Can you work these out from the model? Positions are in its coordinate system, mm. Give positions to 0.01 mm unless a question says otherwise; leave off trailing zeros. Write each loop counter-clockwise with the first axis right and the second up, starting at its lowest first coordinate (ties: lowest second). Pieces come first, ordered by that corner, then holes.
```python
from build123d import *

# Parameters (mm, degrees)
BOSS_EXTRUDE1_DEPTH = 5.9944
SKETCH2_R           = 5.08
CUT_EXTRUDE1_DEPTH  = 369.278830147
CUT_EXTRUDE2_DEPTH  = 1.27
FILLET1_R           = 6.35


with BuildPart() as part:
    # Sketch1 → Boss-Extrude1 (new body)
    with BuildSketch(Plane(origin=(0, 0, 0), x_dir=(1, 0, 0), z_dir=(0, 1, 0))):
        Polygon((-67.6275, 0), (67.6275, 0), (95.613826947, -355.6), (-95.613826947, -355.6), align=None)
    extrude(amount=BOSS_EXTRUDE1_DEPTH)

    # Sketch2 → Cut-Extrude1 (cut, through all)
    with BuildSketch(Plane(origin=(0, 5.9944, 0), x_dir=(1, 0, 0), z_dir=(0, 1, 0))):
        with Locations(Location((0, -101.6, 0), (0, 0, 270))):
            Circle(SKETCH2_R)
    extrude(amount=-CUT_EXTRUDE1_DEPTH, mode=Mode.SUBTRACT)

    # Sketch3 → Cut-Extrude2 (cut)
    # profile 1 of 2: a face of its own
    with BuildSketch(Plane(origin=(0, 5.9944, 0), x_dir=(1, 0, 0), z_dir=(0, 1, 0))):
        Polygon((-0.64745098, -123.339411765), (-2.041960784, -123.339411765), (-2.041960784, -125.73), (-2.838823529, -125.73), (-2.838823529, -123.339411765), (-7.420784314, -123.339411765), (-7.420784314, -122.54254902), (-2.676960784, -115.769215686), (-2.041960784, -115.769215686), (-2.041960784, -122.54254902), (-0.64745098, -122.54254902), align=None)
        Polygon((-2.838823529, -122.54254902), (-2.838823529, -117.185514706), (-6.589681373, -122.54254902), align=None, mode=Mode.SUBTRACT)
    # profile 2 of 2: a face of its own
    with BuildSketch(Plane(origin=(0, 5.9944, 0), x_dir=(1, 0, 0), z_dir=(0, 1, 0))):
        with BuildLine():
            add(Edge.make_bspline(
                [(7.321176471, -120.755833333), (7.318828398, -120.964435203), (7.314268428, -121.369541156), (7.278053355, -121.956745016), (7.212590307, -122.503235643), (7.123658685, -123.008755237), (7.008266172, -123.474678786), (6.871087333, -123.902056716), (6.702092819, -124.287425995), (6.508215245, -124.632617465), (6.291747836, -124.939879658), (6.045192851, -125.205053414), (5.774903263, -125.430333986), (5.47658793, -125.612983557), (5.154255704, -125.75891836), (4.803074469, -125.854617169), (4.428855706, -125.921386338), (4.17035965, -125.926554175), (4.037230392, -125.929215686)],
                knots=[0, 0, 0, 0, 1.444951835, 2.806104229, 4.07292158, 5.255788138, 6.359234241, 7.395665143, 8.361159583, 9.268708362, 10.134304339, 10.95819393, 11.769860228, 12.563733626, 13.374508403, 14.211708464, 15.079003648, 16, 16, 16, 16], degree=3))
            add(Edge.make_bspline(
                [(4.037230392, -125.929215686), (3.904173743, -125.926129436), (3.644961099, -125.920116997), (3.27017657, -125.859085315), (2.920411161, -125.763594373), (2.59640029, -125.625895969), (2.300139806, -125.446021212), (2.024069589, -125.233082993), (1.778627689, -124.975727427), (1.560171839, -124.679785297), (1.365195047, -124.347714828), (1.20253453, -123.973246068), (1.058366082, -123.562916679), (0.945634561, -123.112374896), (0.854092493, -122.625055928), (0.795691583, -122.097466824), (0.752427723, -121.531621273), (0.748884772, -121.140869167), (0.747058824, -120.939485294)],
                knots=[0, 0, 0, 0, 0.942187573, 1.835510922, 2.682899358, 3.50644207, 4.321041037, 5.132947656, 5.970162763, 6.831912057, 7.734836617, 8.692673853, 9.720484412, 10.813675431, 11.980358204, 13.231647047, 14.573260056, 16, 16, 16, 16], degree=3))
            add(Edge.make_bspline(
                [(0.747058824, -120.939485294), (0.749189738, -120.709081181), (0.753301018, -120.264550974), (0.791785956, -119.623892076), (0.848921011, -119.033607435), (0.931327178, -118.493626742), (1.041809864, -118.002956136), (1.18209133, -117.562748274), (1.344352733, -117.168906906), (1.542969603, -116.826611164), (1.76640963, -116.527719309), (2.011736134, -116.265404707), (2.288722816, -116.05041743), (2.588716504, -115.873144616), (2.914180915, -115.735469097), (3.266151279, -115.640569114), (3.642854433, -115.578856283), (3.90312556, -115.573011518), (4.037230392, -115.57)],
                knots=[0, 0, 0, 0, 1.545108237, 2.981054794, 4.302900454, 5.52134946, 6.64223763, 7.672189641, 8.617001291, 9.493094031, 10.318410963, 11.115795503, 11.893970542, 12.661367534, 13.447190288, 14.255881535, 15.101342067, 16, 16, 16, 16], degree=3))
            add(Edge.make_bspline(
                [(4.037230392, -115.57), (4.170238627, -115.57448963), (4.428282356, -115.583199774), (4.804192318, -115.642018007), (5.152618043, -115.745772402), (5.478653289, -115.884356647), (5.772542755, -116.073295118), (6.047681503, -116.293496105), (6.289327541, -116.562467111), (6.510315761, -116.867199073), (6.701841879, -117.215226558), (6.869820244, -117.601739646), (7.009467972, -118.029371708), (7.123413066, -118.496780378), (7.21266615, -119.005311375), (7.277684225, -119.552884468), (7.314472673, -120.141074122), (7.318890361, -120.546189931), (7.321176471, -120.755833333)],
                knots=[0, 0, 0, 0, 0.919968977, 1.784793451, 2.622728724, 3.429378823, 4.225844794, 5.031728358, 5.85964663, 6.718105312, 7.630541726, 8.601153045, 9.629202519, 10.737948011, 11.926092541, 13.198121829, 14.550055913, 16, 16, 16, 16], degree=3))
        make_face()
        with BuildLine():
            add(Edge.make_bspline(
                [(6.524313725, -120.768284314), (6.522566947, -120.59082563), (6.519183425, -120.247086842), (6.491882586, -119.747351272), (6.442379883, -119.282006526), (6.374689104, -118.850591154), (6.287787289, -118.454473729), (6.184085269, -118.091152232), (6.054789642, -117.764549081), (5.914753741, -117.468482457), (5.746577036, -117.21145005), (5.563889756, -116.983709924), (5.356631682, -116.79434266), (5.134096525, -116.633668508), (4.887159424, -116.51702345), (4.624573174, -116.42744118), (4.339914631, -116.378499272), (4.144272117, -116.370819959), (4.043455882, -116.366862745)],
                knots=[0, 0, 0, 0, 1.502278276, 2.909924168, 4.234983773, 5.462469173, 6.604815465, 7.666614396, 8.656743616, 9.57599474, 10.43362925, 11.251287335, 12.040715275, 12.803499886, 13.565626727, 14.343386511, 15.146333119, 16, 16, 16, 16], degree=3))
            add(Edge.make_bspline(
                [(4.043455882, -116.366862745), (3.938447052, -116.369409337), (3.734422845, -116.374357173), (3.43835687, -116.425549656), (3.163244621, -116.509328168), (2.90892764, -116.62546025), (2.673837753, -116.772323146), (2.465862577, -116.959962497), (2.272440236, -117.175944485), (2.105615234, -117.430931462), (1.958401995, -117.71853329), (1.838162718, -118.042916058), (1.738143905, -118.401926091), (1.665875136, -118.800267442), (1.610637384, -119.239896883), (1.570198504, -119.724849093), (1.550557152, -120.257632824), (1.546194025, -120.628198528), (1.543921569, -120.82120098)],
                knots=[0, 0, 0, 0, 0.869467109, 1.689308758, 2.480750345, 3.246411928, 4.000153033, 4.767743238, 5.559605047, 6.396624794, 7.284891774, 8.231849658, 9.258192498, 10.369472511, 11.583108734, 12.929054675, 14.400553601, 16, 16, 16, 16], degree=3))
            add(Edge.make_bspline(
                [(1.543921569, -120.82120098), (1.544614632, -120.988289367), (1.54595406, -121.311207558), (1.570315432, -121.778131708), (1.598441181, -122.210377927), (1.645028029, -122.609499828), (1.709082826, -122.979104893), (1.796740701, -123.322117953), (1.902442711, -123.64204798), (2.027679077, -123.937897338), (2.18133626, -124.206925847), (2.364747317, -124.444835267), (2.580966733, -124.649942715), (2.82339308, -124.825742486), (3.097933318, -124.96336255), (3.398653863, -125.062824592), (3.726651153, -125.123356927), (3.95395607, -125.129287098), (4.071470588, -125.132352941)],
                knots=[0, 0, 0, 0, 1.411809826, 2.728490499, 3.95043818, 5.071756233, 6.122676174, 7.117949067, 8.060697316, 8.967954545, 9.828234386, 10.671864258, 11.496693245, 12.338635446, 13.193491276, 14.080783746, 15.007783125, 16, 16, 16, 16], degree=3))
            add(Edge.make_bspline(
                [(4.071470588, -125.132352941), (4.170329033, -125.130072963), (4.364367231, -125.125597848), (4.644218388, -125.069712213), (4.907756322, -124.987576413), (5.148049832, -124.862984482), (5.372323269, -124.710857365), (5.572547405, -124.519087844), (5.758725654, -124.297778208), (5.918122592, -124.036648789), (6.062406119, -123.745178799), (6.186127809, -123.4196766), (6.291039197, -123.06045838), (6.37874373, -122.667596662), (6.4407328, -122.240695517), (6.492645246, -121.781020892), (6.51900758, -121.286348012), (6.522506852, -120.944697746), (6.524313725, -120.768284314)],
                knots=[0, 0, 0, 0, 0.843506666, 1.655625022, 2.429524786, 3.194843558, 3.95975131, 4.737602927, 5.556133668, 6.424576934, 7.344541811, 8.332537572, 9.395844817, 10.540307741, 11.769239909, 13.080349428, 14.492418622, 16, 16, 16, 16], degree=3))
        make_face(mode=Mode.SUBTRACT)
    extrude(amount=-CUT_EXTRUDE2_DEPTH, mode=Mode.SUBTRACT)

    # Fillet1
    fillet1_edges = [part.edges().sort_by_distance(p)[0] for p in [
        (95.613826947, 2.9972, 355.6),
        (-95.613826947, 2.9972, 355.6),
        (-67.6275, 2.9972, 0),
        (67.6275, 2.9972, 0),
    ]]
    fillet(fillet1_edges, radius=FILLET1_R)


solid = part.part
```
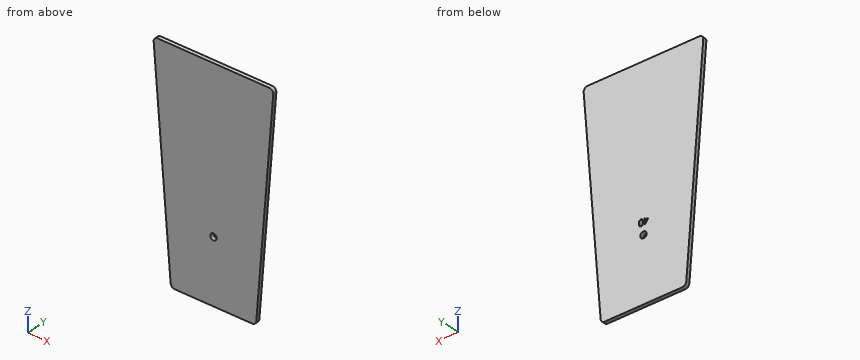
1) Suppose I cut it at A-A on z = 101.6. Write out the boundary of the cut face in (x, y), plus the area to 3 significant figures.
Values follow:
outline: (-75.62, 0) - (-5.08, 0) - (-5.08, 5.99) - (-75.62, 5.99) - close; (5.08, 0) - (75.62, 0) - (75.62, 5.99) - (5.08, 5.99) - close
area: 846 mm2
2) Suppose I cut it at C-C on z = 161. Write out the boundary of the cut face in (x, y).
Values follow:
outline: (-80.3, 0) - (80.3, 0) - (80.3, 5.99) - (-80.3, 5.99) - close
3) For pin 1 Ø1.4 at (y, z) = (5.5, 118) entering from -X; pin 2 Ø2 at (y, z) = (4.5, 234.5) entering from +X; pin 3 Ø9 at (x, z) = (0, 101.6) entering from -Y; pin 4 Ø0.6 at (y, z) = (5, 124.5) entering from +X, each with a flat end and sliding along its axis, tell me the tip position at first contact or that it passes through.
Values follow:
pin 1: stops at x = -76.97
pin 2: stops at x = 86.16
pin 3: passes through
pin 4: stops at x = 77.45
4) Suppose I cut it at B-B on z = 203. Write out the boundary of the cut face in (x, y), plus the area to 3 significant figures.
Values follow:
outline: (-83.6, 0) - (83.6, 0) - (83.6, 5.99) - (-83.6, 5.99) - close
area: 1,000 mm2
5) Please list where these lines run through material, in increasing order: L1, parallel to X at y = 2.25, z = 101.6; L2, parallel to X at y = 3.4, z = 116.5; L3, parallel to X at y = 1.4, z = 180.5.
Values follow:
L1: x = -75.62 to -5.08, 5.08 to 75.62
L2: x = -76.8 to 76.8
L3: x = -81.83 to 81.83
